Part model, mm, in its own coordinate system. A direction names the side the tool comes from. Round coordinates to 2 decimals unless told otherwise and drop trailing zeros. Write each loop counter-clockwise with the first axis right and the second up, starting at its lowest first coordinate (ties: lowest second). Pieces come first, ordered by that corner, then holes. Notation, with made-up numbers: (-3.5, 14) -> (31.5, 14) arc R30 cw to (31.5, 43) -> close; hole circle Ø9 at (88.25, 76). An arc over 180 degrees is marked (long way). Return JSON: item names as keys, results as strings. Group by question number.
(1) Drill centre lines: L1, parallel to Y at x = -15.5, z = 11; L2, parallel to X at y = -99, z = 16.25; L3, parallel to Y at x = -158, z = 2.25. Where is each one in solid material? Low to high. Write a range as from..to.
(2) Saw through at D-D (y = -210). List the corners of the cut face in (x, z), plus the area to 3 significant figures.
(3) Saw through at B-B (x = 27). List the corners of the cut face in (y, z).
(4) Saw through at A-A (y = 73). List the corners of the cut face in (x, z), plus the area to 3 significant figures.
(5) Drop flat-ended pins along their axis: pin 1 Ø10 at (x, z) = (84.5, 14.5) entering from -Y; pin 2 Ø10 at (x, z) = (150.5, 2.5) entering from +Y; pin 3 Ø8 at (x, z) = (98, 16.5) entering from +Y; pin 4 Ø6 at (x, y) = (154.27, -183.85) entering from -Z. Give the stop position or say it passes through.
(6) Tool access for faces 1 (the flat face through (246.423, 42.158, 9.86)), 2 (the flat face through (82.622, -230.652, 12.395)): list every direction of +Z, -Z, +X, -X, +Y, -Y with a clear straight run to the whole face (end or side of a thin tool).
(7) Saw through at C-C (z = 17). State how many separate pieces and enclosed holes the cut face has, plus the area to 3 significant figures.
(8) Mould opens along Y. For faces 3 (the flat face through (-245.98, 44.67, 9.86)), 4 (the cylindrical face through (83.06, -159.69, 12.6)), 5 (the flat face through (-79, -236, 20)) say: +Y half, -Y half, draft (parallel to the pull), parting line (faces both ways), or undercut.
from build123d import *

# Parameters (mm, degrees)
F1_DEPTH = 20
F2_R     = 175
F3_DEPTH = 20.001
F4_R     = 5
F5_DEPTH = 20.001
F6_T     = -5


with BuildPart() as f1:
    # F0 (on Top) → F1 (new body)
    with BuildSketch(Plane.XY):
        Polygon((90.9925585666, 250), (-90.9925585666, 250), (-230.4012462767, 133.0222215595), (-262.0026302294, -46.198132726), (-171.0100716628, -203.801867274), (0, -266.044443119), (171.0100716628, -203.801867274), (262.0026302294, -46.198132726), (230.4012462767, 133.0222215595), align=None)
    extrude(amount=F1_DEPTH)

    # F2 (on face) → F3 (cut, through all)
    with BuildSketch(Plane.XY.offset(20)):
        Circle(F2_R)
    extrude(amount=-F3_DEPTH, mode=Mode.SUBTRACT)

    # F4 (on face) → F5 (cut, through all)
    with BuildSketch(Plane.XY.offset(20)):
        with Locations((-154.2690263248, -183.8506663486)):
            Circle(F4_R)
        with Locations((236.3538607229, -41.6755626401)):
            Circle(F4_R)
        with Locations((82.0848343982, 225.5262289886)):
            Circle(F4_R)
        with Locations((-236.3538607229, -41.6755626401)):
            Circle(F4_R)
        with Locations((154.2690263248, -183.8506663486)):
            Circle(F4_R)
        with Locations((-82.0848343982, 225.5262289886)):
            Circle(F4_R)
    extrude(amount=-F5_DEPTH, mode=Mode.SUBTRACT)

    # F6
    f6_openings = [f1.faces().sort_by_distance(p)[0] for p in [
        (155.969535, 185.877254, 20),
    ]]
    offset(amount=F6_T, openings=f6_openings)


solid = f1.part
Computed values:
{
 "1": {"L1": "-260.4..-255.08, -179.33..-174.31, 174.31..179.33, 245..250", "L2": "-231.52..-225.74, -150.33..-144.31, 144.31..150.33, 225.74..231.52", "L3": "-208.54..-187.18, -180.52..-75.24, 75.24..193.77"},
 "2": {"outline": "(-153.98, 0) -> (153.98, 0) -> (153.98, 20) -> (139.36, 20) -> (139.36, 5) -> (-139.36, 5) -> (-139.36, 20) -> (-153.98, 20) -> close", "area": "1,980 mm2"},
 "3": {"outline": "(-256.22, 0) -> (-172.9, 0) -> (-172.9, 20) -> (-177.96, 20) -> (-177.96, 5) -> (-250.9, 5) -> (-250.9, 20) -> (-256.22, 20) -> close; (172.9, 0) -> (250, 0) -> (250, 20) -> (245, 20) -> (245, 5) -> (177.96, 5) -> (177.96, 20) -> (172.9, 20) -> close"},
 "4": {"outline": "(-240.98, 0) -> (-159.05, 0) -> (-159.05, 20) -> (-164.53, 20) -> (-164.53, 5) -> (-235.91, 5) -> (-235.91, 20) -> (-240.98, 20) -> close; (159.05, 0) -> (240.98, 0) -> (240.98, 20) -> (235.91, 20) -> (235.91, 5) -> (164.53, 5) -> (164.53, 20) -> (159.05, 20) -> close", "area": "1,140 mm2"},
 "5": {"pin 1": "y = -237.11", "pin 2": "y = 204.26", "pin 3": "y = 247.48", "pin 4": "through"},
 "6": {"face 1": "+Z, -Z, +X, +Y", "face 2": "+Z"},
 "7": {"separate pieces": "8", "enclosed holes": "8", "area": "15,100 mm2"},
 "8": {"face 3": "+Y half", "face 4": "undercut", "face 5": "draft"}
}
